Design review of the part shown in the three views and the two pictorial views. Dimensions are in mm from the part's minimum x, y and z. A direction names the side the tool comes from. Coordinates: 2 decimals unless noted, no trailing zeros. Write each loop counter-clockwise with the first axis right and the second up, starting at its lowest first coordinate (ties: lowest second). Pieces come first, ordered by that corner, then holes. Notation, with made-up numbers: (-17, 47) -> (7, 47) arc R21 ccw to (7, 77) -> close; hole circle Ø6 at (-8.75, 21.5). An arc over 180 degrees is marked (long way). Answer in a Markdown table with one row per item. Add a question column.
Item 1: Take a section at C-C, the plane x = 5. Write out the cut boundary in (y, z), and give its area (3 significant figures).
Item 2: Take a section at A-A, the plane z = 43. Write out the cut boundary in (x, y), and give its area (3 significant figures).
Item 3: Draft analysis for pull direction Z (two halves, no side actions). For the marked faces 1, 2 and 3, state which applies: released by +Z, released by -Z, zero draft, split by the parting line, or undercut.
Item 4: Take a section at D-D, the plane z = 24. Write out the cut boundary in (x, y), and give its area (3 significant figures).
Item 5: To check wall thickness, follow line 1 (X direction, y = 0.7, z = 5); line 2 (Z direction, x = 23, y = 1.75); line 3 (Z direction, x = 32, y = 15.5). State the ranges of each line that lie inside material, in increasing order.
Item 6: Take a section at B-B, the plane y = 4.75. Write out the cut boundary in (x, z), and give its area (3 significant figures).
Item 7: Clearance check with flat-ended pins moving along their axes: P1, Ø2, axis at x = 25, z = 11, coming from the +Y side; P2, Ø4, axis at x = 30, y = 13, coming from the -Z side; P3, Ø4.5, axis at y = 19, z = 20, coming from the +X side; P4, Ø2.5, axis at x = 5, z = 43, coming from the +Y side. State where each tip first meets the part, or that it passes through.
Item 8: For the marked faces 4, 5, 6, 7 and 8, list the 3-axis set-ups (+Z, -Z, +X, -X, +Y, -Y) from which the entire face can be reached by the end or side of a thin tool; tool diameter is ignored.
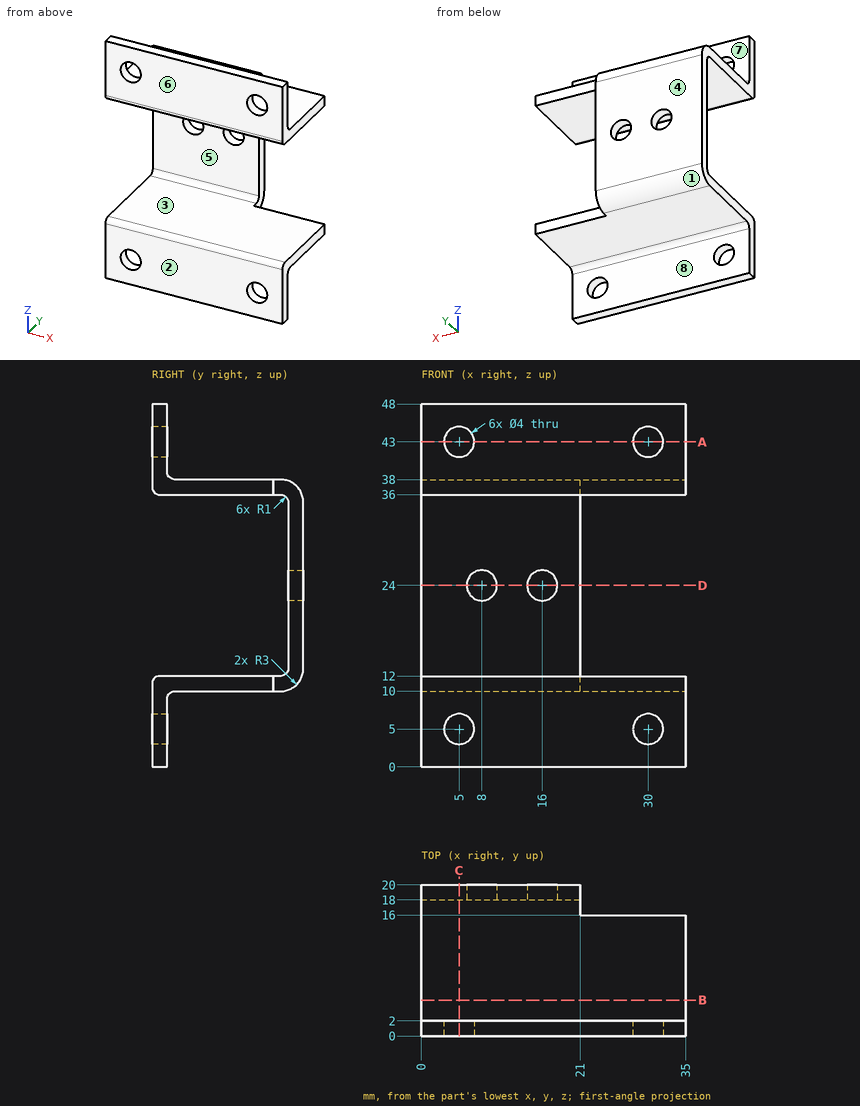
Answers:
| question | item | result |
|---|---|---|
| 1 | outline | (0, 0) -> (2, 0) -> (2, 3) -> (0, 3) -> close; (0, 7) -> (2, 7) -> (2, 9) arc R1 cw to (3, 10) -> (17, 10) arc R3 ccw to (20, 13) -> (20, 35) arc R3 ccw to (17, 38) -> (3, 38) arc R1 cw to (2, 39) -> (2, 41) -> (0, 41) -> (0, 37) arc R1 ccw to (1, 36) -> (17, 36) arc R1 cw to (18, 35) -> (18, 13) arc R1 cw to (17, 12) -> (1, 12) arc R1 ccw to (0, 11) -> close; (0, 45) -> (2, 45) -> (2, 48) -> (0, 48) -> close |
| 1 | area | 149 mm^2 |
| 2 | outline | (0, 0) -> (3, 0) -> (3, 2) -> (0, 2) -> close; (7, 0) -> (28, 0) -> (28, 2) -> (7, 2) -> close; (32, 0) -> (35, 0) -> (35, 2) -> (32, 2) -> close |
| 2 | area | 54.0 mm^2 |
| 3 | face 1 | released by -Z |
| 3 | face 2 | zero draft |
| 3 | face 3 | undercut |
| 4 | outline | (0, 18) -> (6, 18) -> (6, 20) -> (0, 20) -> close; (10, 18) -> (14, 18) -> (14, 20) -> (10, 20) -> close; (18, 18) -> (21, 18) -> (21, 20) -> (18, 20) -> close |
| 4 | area | 26.0 mm^2 |
| 5 | line 1 | x = 0 to 3, 7 to 28, 32 to 35 |
| 5 | line 2 | z = 0 to 12, 36 to 48 |
| 5 | line 3 | z = 10 to 12, 36 to 38 |
| 6 | outline | (0, 10) -> (35, 10) -> (35, 12) -> (0, 12) -> close; (0, 36) -> (35, 36) -> (35, 38) -> (0, 38) -> close |
| 6 | area | 140 mm^2 |
| 7 | P1 | stops at y = 16 |
| 7 | P2 | stops at z = 10 |
| 7 | P3 | stops at x = 21 |
| 7 | P4 | passes through |
| 8 | face 4 | +Z, -Z, +X, -X, +Y |
| 8 | face 5 | +X, -X, -Y |
| 8 | face 6 | +Z, -Z, +X, -X, -Y |
| 8 | face 7 | +Z, +X, -X, +Y |
| 8 | face 8 | -Z, +X, -X, +Y |
